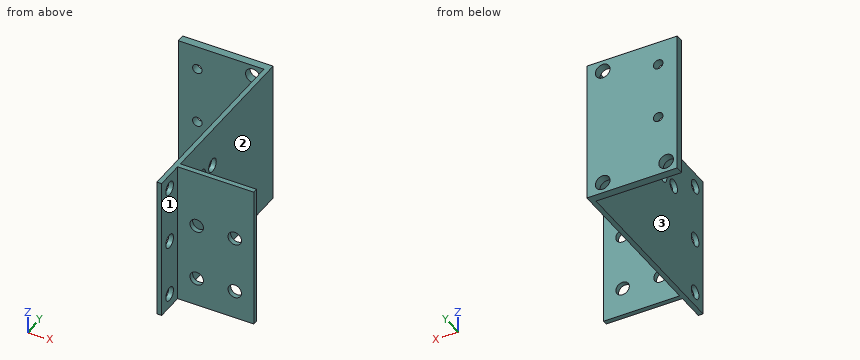
Autodesk Inventor part; units mm, degrees
ref_plane "YZ Plane" through (0, 0, 0) normal (1, 0, 0) x (0, 1, 0)
ref_plane "XZ Plane" through (0, 0, 0) normal (0, 1, 0) x (-1, 0, 0)
ref_plane "XY Plane" through (0, 0, 0) normal (0, 0, 1) x (1, 0, 0)
sketch "Sketch3" plane through (0, 0, 0) normal (0, 1, 0) x (-1, 0, 0)
  line L0 (0, 0) -> (27, 0)
  line L1 (27, 0) -> (27, -45)
  line L2 (27, -45) -> (0, -45)
  line L3 (0, -45) -> (0, 0)
  dimension "d27" = 27
  dimension "d28" = 45
extrude "Extrusion2" add sketch "Sketch3" along normal blind 2.5
sketch "Sketch4" plane through (0, 0, 0) normal (0, -1, 0) x (1, 0, 0)
  line L0 (0, 0) -> (1.5, 0)
  line L1 (1.5, 0) -> (1.5, -45)
  line L2 (1.5, -45) -> (0, -45)
  line L3 (0, -45) -> (0, 0)
  dimension "d31" = 1.5
  dimension "d32" = 45
extrude "Extrusion3" add sketch "Sketch4" along normal blind 60 and the other way blind 2.5
sketch "Sketch5" plane through (0, 2.5, 0) normal (0, 1, 0) x (1, 0, 0)
  line L0 (-27, 0) -> (-27, 45)
  line L1 (-27, 0) -> (1.5, 0)
  circle A0 centre (-3.5, 3.5) radius 2.3
  line L2 (0, 45) -> (0, 0)
  circle A1 centre (-23.5, 41.5) radius 2.3
  line L3 (1.5, 45) -> (-27, 45)
  circle A2 centre (-3.5, 41.5) radius 2.3
  dimension "d45" = 4.6
  dimension "d46" = 3.5
  dimension "d47" = 3.5
  dimension "d50" = 4.6
  dimension "d51" = 3.5
  dimension "d52" = 4.6
  dimension "d61" = 3.5
  dimension "d62" = 3.5
  dimension "d63" = 3.5
hole "Hole2" at (-3.5, 2.5, -3.5) at (-3.5, 2.5, -41.5) at (-23.5, 2.5, -41.5) direction (0, -1, 0) diameter 4.6 end through all
sketch "Sketch6" plane through (0, 2.5, 0) normal (0, 1, 0) x (1, 0, 0)
  circle A0 centre (-21, 7.5) radius 1.5
  line L0 (-27, 45) -> (-27, 0)
  line L1 (-27, 0) -> (1.5, 0)
  circle A1 centre (-21, 25.5) radius 1.5
  point P0 (0, 0)
  dimension "d64" = 3
  dimension "d65" = 6
  dimension "d66" = 7.5
  dimension "d67" = 3
  dimension "d68" = 18
hole "Hole3" at (-21, 2.5, -7.5) at (-21, 2.5, -25.5) direction (0, -1, 0) diameter 3 end through all
sketch "Sketch7" plane through (1.5, -60, 0) normal (1, 0, 0) x (0, 0, -1)
  circle A0 centre (4.5, 4.5) radius 2.15
  line L0 (45, 0) -> (0, 0)
  line L1 (0, 0) -> (0, 62.5)
  circle A1 centre (40.5, 4.5) radius 2.15
  line L2 (45, 0) -> (45, 62.5)
  circle A2 centre (22.5, 4.5) radius 2.15
  point P0 (0, 60)
  dimension "d76" = 4.3
  dimension "d77" = 4.5
  dimension "d78" = 4.5
  dimension "d79" = 4.3
  dimension "d80" = 4.5
  dimension "d81" = 4.5
  dimension "d82" = 4.3
hole "Hole4" at (1.5, -55.5, -4.5) at (1.5, -55.5, -22.5) at (1.5, -55.5, -40.5) direction (-1, 0, 0) diameter 4.3 end through all
sketch "Sketch8" plane through (1.5, -60, 0) normal (1, 0, 0) x (0, 0, -1)
  line L0 (0, 9) -> (45, 9)
  line L1 (45, 9) -> (45, 10.5)
  line L2 (45, 10.5) -> (0, 10.5)
  line L3 (0, 10.5) -> (0, 9)
  line L4 (0, 62.5) -> (45, 62.5)
  point P0 (0, 60)
  dimension "d90" = 45
  dimension "d91" = 1.5
  dimension "d92" = 52
extrude "Extrusion4" add sketch "Sketch8" along normal blind 24
sketch "Sketch10" plane through (1.5, -49.5, 0) normal (0, 1, 0) x (1, 0, 0)
  circle A0 centre (6, 36) radius 2.125
  line L0 (0, 45) -> (24, 45)
  line L1 (0, 0) -> (0, 45)
  circle A1 centre (18, 36) radius 2.125
  line L2 (6, 36) -> (6, 27)
  line L3 (6, 27) -> (12, 27)
  circle A2 centre (6, 18) radius 2.125
  circle A3 centre (18, 18) radius 2.125
  point P0 (-1.5, 0)
  dimension "d95" = 4.25
  dimension "d96" = 9
  dimension "d97" = 6
  dimension "d100" = 4.25
  dimension "d102" = 9
hole "Hole6" at (7.5, -49.5, -18) at (7.5, -49.5, -36) at (19.5, -49.5, -36) at (19.5, -49.5, -18) direction (0, -1, 0) diameter 4.25 end through all
sketch "Sketch11" plane through (1.5, 2.5, 0) normal (1, 0, 0) x (0, 0, -1)
  circle A0 centre (12, -46) radius 2.125
  line L0 (45, -52) -> (45, 0)
  line L1 (0, -52) -> (0, 0)
  line L2 (0, -52) -> (45, -52)
  circle A1 centre (12, -40) radius 2.125
  circle A2 centre (12, -34) radius 2.125
  point P0 (0, -2.5)
  dimension "d117" = 4.25
  dimension "d119" = 12
  dimension "d120" = 6
  dimension "d121" = 4.25
  dimension "d122" = 6
  dimension "d123" = 4.25
  dimension "d124" = 6
hole "Hole7" at (1.5, -31.5, -12) at (1.5, -37.5, -12) at (1.5, -43.5, -12) direction (-1, 0, 0) diameter 4.25 depth 8 tip angle 118
properties part number "TrolleyRightPlate"
Geometry check sheet. Reference: the model listing, model coordinates, mm. Face numbers are marked on the shaded views. A direction names the side the tool comes from. Give positions to 0.01 mm unless a question says otherwise; leave off trailing zeros. Write each loop counter-clockwise with the first axis right and the second up, starting at its lowest first coordinate (ties: lowest second). Pieces come first, ordered by that corner, then holes. Notation, with made-up numbers: M 27.25,1 L 62.25,1 A28 cw 62.25,19 Z; hole C 1.25,3.25 d7. An arc over 180 degrees is marked long. Answer as CSV lines item,"result". Start each with the question number.
Q1. Tool access check on the marked faces 1, 2 and 3. Record the directions out of +Z, -Z, +X, -X, +Y, -Y that give a thin tool (end or side, any length) a straight path to the whole face; none if there is none.
Q2. Go/stop test with flat-tipped pins: pin 1 (12 mm diameter, centred on x = 20, z = -11.5, fed in from -Y); pin 2 (5 mm diameter, centred on y = -55.5, z = -22.5, fed in from -X); pin 3 (12 mm diameter, centred on x = -9.5, z = -40.5, fed in from -Y); pin 4 (7.5 mm diameter, centred on x = -3.5, z = -3.5, fed in from +Y). Record where each tip stops, or that it passes through.
Q3. Section check C-C, the plane x = 19.5. Record the cut outline in (y, z) (3 decimals).
Q4. Section check B-B, the plane z = -36. Record the cut outline in (x, y) (3 decimals).
Q5. Section check D-D, the plane z = -8. Record the cut outline in (x, y).
Q6. Section check A-A, the plane y = -43.5. Record the cut outline in (x, z) (3 decimals), then the cut area to 3 significant figures.
Q7. Material ranges on L1, parallel to X at y = 1.5, z = -41.5; L2, parallel to Z at x = -3.5, y = 0.7; L3, parallel to Z at x = 0.3, y = -55.5, recorded low to high.
Geometry says:
1,face 1,"+Z, -Z, +X, -Y"
1,face 2,"+Z, -Z, +X, +Y"
1,face 3,"+Z, -Z, -X, -Y"
2,pin 1,"y = -51"
2,pin 2,"x = 0"
2,pin 3,"y = 0"
2,pin 4,"y = 2.5"
3,outline,"M -51,-45 L -49.5,-45 L -49.5,-38.125 L -51,-38.125 Z; M -51,-33.875 L -49.5,-33.875 L -49.5,-20.125 L -51,-20.125 Z; M -51,-15.875 L -49.5,-15.875 L -49.5,0 L -51,0 Z"
4,outline,"M -27,0 L 0,0 L 0,-60 L 1.5,-60 L 1.5,-51 L 5.375,-51 L 5.375,-49.5 L 1.5,-49.5 L 1.5,2.5 L -27,2.5 Z; M 9.625,-51 L 17.375,-51 L 17.375,-49.5 L 9.625,-49.5 Z; M 21.625,-51 L 25.5,-51 L 25.5,-49.5 L 21.625,-49.5 Z"
5,outline,"M -27,0 L -22.41,0 L -22.41,2.5 L -27,2.5 Z; M -19.59,0 L 0,0 L 0,-60 L 1.5,-60 L 1.5,-51 L 25.5,-51 L 25.5,-49.5 L 1.5,-49.5 L 1.5,2.5 L -19.59,2.5 Z"
6,outline,"M 0,-45 L 1.5,-45 L 1.5,-14.125 L 0,-14.125 Z; M 0,-9.875 L 1.5,-9.875 L 1.5,0 L 0,0 Z"
6,area,"61.1 mm^2"
7,L1,"-27 to -25.8, -21.2 to -5.8, -1.2 to 1.5"
7,L2,"-45 to -43.8, -39.2 to -5.8, -1.2 to 0"
7,L3,"-45 to -42.65, -38.35 to -24.65, -20.35 to -6.65, -2.35 to 0"
